Design review of the part built by this model. Coordinates are the model's own, in mm. Coordinates: 2 decimals unless noted, no trailing zeros. Loops run counter-clockwise (first coordinate to the right, second up) from the corner with the lowest first, then second, coordinate; pieces in that order, holes last. Notation, with made-up numbers: (80.5, 43.25) -> (121.5, 43.25) arc R25 cw to (121.5, 73.25) -> close; hole circle Ø2 at (65.25, 37.5). An arc over 180 degrees is marked (long way). Use a Markdown table: item, result. Add a question column.
Q1. Take a section at B-B on z = 0. Write out the cut boundary in (x, y), plus the area to 3 significant figures.
Q2. Draft analysis for pull direction Y (two halves, no side actions). For faces 1 (the face through (0, 4, 2)), 2 (the face through (1, 6, 1)), 3 (the face through (-1.5, 0.99, -0.07)), state which applies: pulls with the +Y half, pulls with the -Y half, needs draft (parallel to the pull), parting line crosses it, or undercut.
Q3. Take a section at C-C on y = 5.75. Write out the cut boundary in (x, z), plus the area to 3 significant figures.
Q4. Clearance check with flat-ended pins moving along their axes: pin 1 Ø1 at (x, y) = (-1.5, -3) entering from +Z; pin 2 Ø2 at (x, y) = (-1.5, 2.5) entering from +Z. State where each tip first meets the part, or that it passes through.
Q5. Take a section at A-A on x = 0. Write out the cut boundary in (y, z), plus the area to 3 significant figures.
Q6. Take a section at D-D on z = 1.3. Write out the cut boundary in (x, y).
Q7. For probe 1 along Z at (x, y) = (0, -2.5); probe 2 along Y at (x, z) = (-0.95, -1.65), list the stretches that pass through material, from the lowest coordinate up.
from build123d import *

# Parameters (mm, degrees)
SKETCH_1_R           = 2
SKETCH_1_R_2         = 1
EXTRUDE_1_DEPTH      = 6
EXTRUDE_1_DEPTH_BACK = 4
SKETCH_2_R           = 2
SKETCH_2_R_2         = 1.5
CUT_EXTRUDE_1_DEPTH  = 2


with BuildPart() as part:
    # 草图1 → 凸台-拉伸1 (new body, two sides)
    with BuildSketch(Plane(origin=(0, 0, 0), x_dir=(1, 0, 0), z_dir=(0, 1, 0))) as extrude_1_sk:
        Circle(SKETCH_1_R)
        Circle(SKETCH_1_R_2, mode=Mode.SUBTRACT)
    extrude(amount=EXTRUDE_1_DEPTH)
    extrude(extrude_1_sk.sketch, amount=-EXTRUDE_1_DEPTH_BACK)

    # 草图2 → 切除-拉伸1 (cut)
    with BuildSketch(Plane(origin=(0, 0, 0), x_dir=(1, 0, 0), z_dir=(0, 1, 0))):
        Circle(SKETCH_2_R)
        Circle(SKETCH_2_R_2, mode=Mode.SUBTRACT)
    extrude(amount=CUT_EXTRUDE_1_DEPTH, mode=Mode.SUBTRACT)


solid = part.part
Answer list:
| question | item | result |
|---|---|---|
| 1 | outline | (-2, -4) -> (-1, -4) -> (-1, 6) -> (-2, 6) -> (-2, 2) -> (-1.5, 2) -> (-1.5, 0) -> (-2, 0) -> close; (1, -4) -> (2, -4) -> (2, 0) -> (1.5, 0) -> (1.5, 2) -> (2, 2) -> (2, 6) -> (1, 6) -> close |
| 1 | area | 18.0 mm² |
| 2 | face 1 | needs draft |
| 2 | face 2 | pulls with the +Y half |
| 2 | face 3 | undercut |
| 3 | outline | circle Ø4 at (0, 0); hole circle Ø2 at (0, 0) |
| 3 | area | 9.42 mm² |
| 4 | pin 1 | z = 1.73 |
| 4 | pin 2 | z = 1.94 |
| 5 | outline | (-4, -2) -> (0, -2) -> (0, -1.5) -> (2, -1.5) -> (2, -2) -> (6, -2) -> (6, -1) -> (-4, -1) -> close; (-4, 1) -> (6, 1) -> (6, 2) -> (2, 2) -> (2, 1.5) -> (0, 1.5) -> (0, 2) -> (-4, 2) -> close |
| 5 | area | 18.0 mm² |
| 6 | outline | (-1.52, -4) -> (1.52, -4) -> (1.52, 0) -> (0.75, 0) -> (0.75, 2) -> (1.52, 2) -> (1.52, 6) -> (-1.52, 6) -> (-1.52, 2) -> (-0.75, 2) -> (-0.75, 0) -> (-1.52, 0) -> close |
| 7 | probe 1 | -2 to -1, 1 to 2 |
| 7 | probe 2 | -4 to 0, 2 to 6 |
